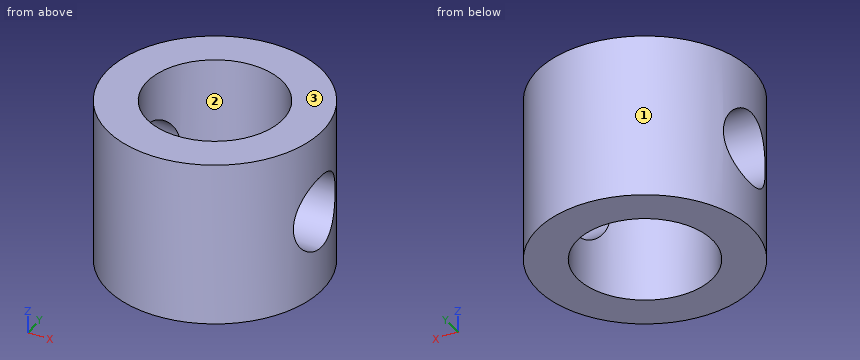
from build123d import *

# Parameters (mm, degrees)
F0_R     = 6.5
F1_DEPTH = 10
F2_R     = 4.1
F3_DEPTH = 10
F4_R     = 2.25
F5_DEPTH = 12.5


with BuildPart() as f1:
    # F0 (on Top) → F1 (new body)
    with BuildSketch(Plane.XY):
        Circle(F0_R)
    extrude(amount=F1_DEPTH)

    # F2 (on face) → F3 (cut)
    with BuildSketch(Plane.XY.offset(10)):
        Circle(F2_R)
    extrude(amount=-F3_DEPTH, mode=Mode.SUBTRACT)

    # F4 (on Right) → F5 (cut, symmetric)
    with BuildSketch(Plane.YZ):
        with Locations((0, 5)):
            Circle(F4_R)
    extrude(amount=F5_DEPTH, both=True, mode=Mode.SUBTRACT)


solid = f1.part
Could you check a few things on this model? Use its own coordinates, in mm. Face numbers are marked on the shaded views. Coordinates: 2 decimals unless noted, no trailing zeros. Write each loop counter-clockwise with the first axis right and the second up, starting at its lowest first coordinate (ties: lowest second). Pieces come first, ordered by that corner, then holes. Notation, with made-up numbers: (80, 36.5) - (110, 36.5) arc R31 cw to (110, 60.5) - close; hole circle Ø1 at (37.25, -32.5). An arc over 180 degrees is marked (long way). Put each result on its own line as item: value. Start each with the question number.
Q1. I want a section at A-A on x = 0. Write out the boundary of the cut face in (y, z), plus the area to 3 significant figures.
Q2. Thinking about a two-plate mould opening in Y: for the marked faces 1, 2 and 3, which applies, pulls with the +Y half, pulls with the -Y half, needs draft (parallel to the pull), parting line crosses it, or undercut?
Q3. I'm going to push flat-ended pins straight in: P1, Ø1, axis at x = -5, z = 8.5, coming from the -Y side; P2, Ø1, axis at y = -5, z = 5.5, coming from the +X side; P3, Ø2, axis at y = -5, z = 4.5, coming from the +X side. Where does each tip first touch, or does it pass through?
Q4. Please list where these lines run through material, in increasing order: L1, parallel to Y at x = 0, z = 6; L2, parallel to Y at x = 1.5, z = 6.75; L3, parallel to X at y = -1, z = 7.25.
Q5. I want a section at B-B on y = 3.5. Write out the boundary of the cut face in (x, z).
Q6. I want a section at C-C on y = 0. Write out the boundary of the cut face in (x, z), plus the area to 3 significant figures.
Q7. I want a section at D-D on z = 2. Write out the boundary of the cut face in (x, y).
Checks:
1. outline: (-6.5, 0) - (-4.1, 0) - (-4.1, 10) - (-6.5, 10) - close; (4.1, 0) - (6.5, 0) - (6.5, 10) - (4.1, 10) - close
1. area: 48.0 mm²
2. face 1: parting line crosses it
2. face 2: undercut
2. face 3: needs draft
3. P1: y = -4.69
3. P2: x = 4.69
3. P3: x = 5.12
4. L1: -6.5 to -4.1, 4.1 to 6.5
4. L2: -6.32 to -3.82, 3.82 to 6.32
4. L3: -6.42 to -3.98, 3.98 to 6.42
5. outline: (-5.48, 0) - (-2.14, 0) - (-2.14, 10) - (-5.48, 10) - close; (2.14, 0) - (5.48, 0) - (5.48, 10) - (2.14, 10) - close
6. outline: (-6.5, 0) - (-4.1, 0) - (-4.1, 2.75) - (-6.5, 2.75) - close; (-6.5, 7.25) - (-4.1, 7.25) - (-4.1, 10) - (-6.5, 10) - close; (4.1, 0) - (6.5, 0) - (6.5, 2.75) - (4.1, 2.75) - close; (4.1, 7.25) - (6.5, 7.25) - (6.5, 10) - (4.1, 10) - close
6. area: 26.4 mm²
7. outline: circle Ø13 at (0, 0); hole circle Ø8.2 at (0, 0)
